Input: dimensioned drawing with shaded views. Units: mm. Origin: part minimum x, y, z. Coordinates: 2 decimals unless noted, no trailing zeros. Loops run counter-clockwise (first coordinate to the right, second up) from the corner with the lowest first, then second, coordinate; pieces in that order, holes last.
Item 1: Section A-A on z = 17.75. Give the number of separate pieces and of enclosed holes in the cut face.
Item 2: Ray query, line 1 along X through (y, z) = (2, 18.9); line 2 along X through (y, z) = (20.5, 19.75); line 3 along Z through (x, y) = (1.3, 37). Return the intervals inside material, ascending.
Item 3: Contact query for a flat-ended pin moving along its axis: P1, Ø1.5, axis at x = 1.5, y = 13.5, coming from the +Z side. Output: stop coordinate, or through.
Item 4: Section C-C on y = 24.5. Return loops of the section in (x, z).
Item 5: Section B-B on y = 48. Return loops of the section in (x, z).
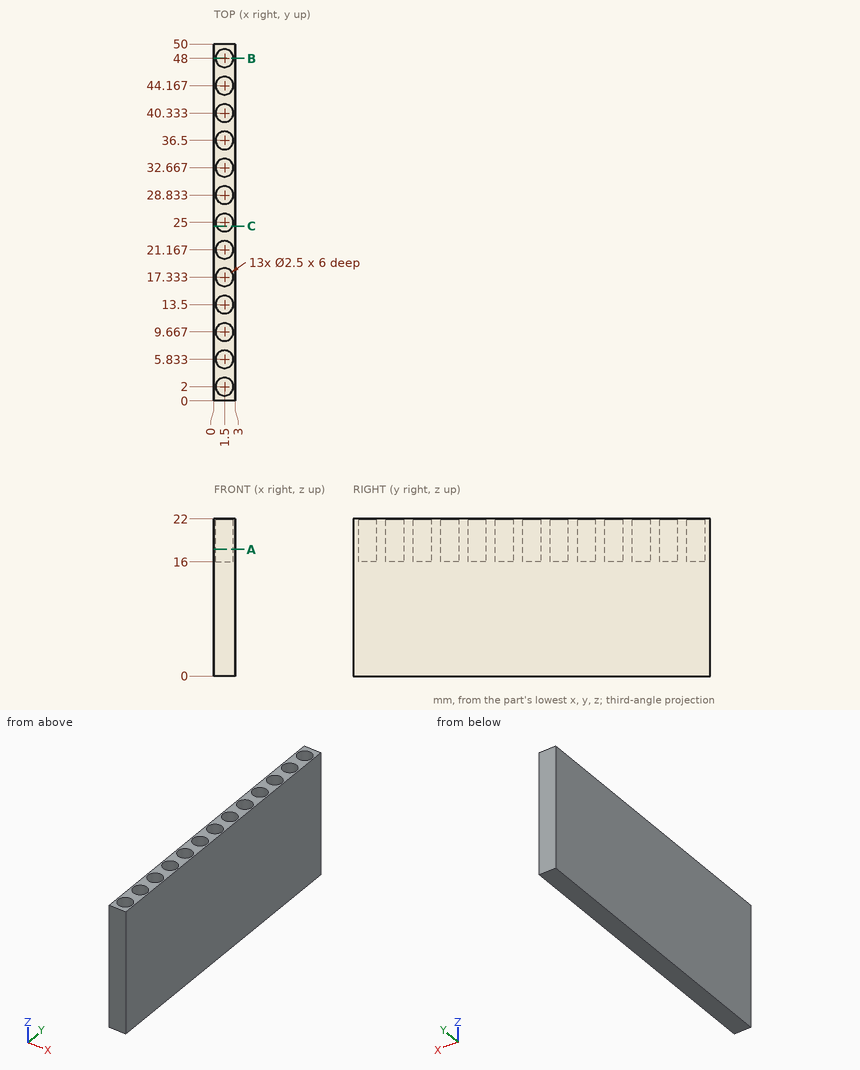
Results found:
1. separate pieces: 1
1. enclosed holes: 13
2. line 1: x = 0 to 0.25, 2.75 to 3
2. line 2: x = 0 to 0.44, 2.56 to 3
2. line 3: z = 0 to 16
3. P1: stops at z = 16
4. outline: (0, 0) - (3, 0) - (3, 22) - (2.65, 22) - (2.65, 16) - (0.35, 16) - (0.35, 22) - (0, 22) - close
5. outline: (0, 0) - (3, 0) - (3, 22) - (2.75, 22) - (2.75, 16) - (0.25, 16) - (0.25, 22) - (0, 22) - close
